Autodesk Inventor part; units mm, degrees
ref_plane "YZ Plane" through (0, 0, 0) normal (1, 0, 0) x (0, 1, 0)
ref_plane "XZ Plane" through (0, 0, 0) normal (0, 1, 0) x (-1, 0, 0)
ref_plane "XY Plane" through (0, 0, 0) normal (0, 0, 1) x (1, 0, 0)
sketch "Sketch1" plane through (0, 0, 0) normal (0, 1, 0) x (-1, 0, 0)
  line L0 (0, 0) -> (85.6, 0)
  line L1 (85.6, 0) -> (85.6, 53.98)
  line L2 (85.6, 53.98) -> (0, 53.98)
  line L3 (0, 53.98) -> (0, 0)
  line L4 (0, 53.98) -> (0, 50.8)
  line L5 (0, 50.8) -> (3.18, 50.8)
  circle A0 centre (3.18, 50.8) radius 3.18
  line L6 (85.6, 53.98) -> (85.6, 57.98)
  line L7 (85.6, 57.98) -> (0, 57.98)
  line L8 (0, 57.98) -> (-9, 57.98)
  line L9 (-9, 57.98) -> (-9, 0)
  line L10 (-9, 0) -> (0, 0)
  line L11 (0, 26.99) -> (-4.5, 26.99)
  circle A1 centre (-4.5, 26.99) radius 2.5
  line L12 (85.6, 55.98) -> (65.6, 55.98)
  circle A2 centre (65.6, 55.98) radius 1
  line L13 (0, 26.99) -> (85.6, 26.99)
  line L14 (85.6, -4) -> (0, -4)
  line L15 (0, -4) -> (-9, -4)
  circle A3 centre (65.6, -2) radius 1
  line L16 (85.6, -4) -> (85.6, 0)
  line L17 (-9, -4) -> (-9, 0)
  line L18 (85.6, 57.98) -> (88.6, 57.98)
  line L19 (88.6, 57.98) -> (88.6, -4)
  line L20 (88.6, -4) -> (85.6, -4)
  line L21 (85.6, -4) -> (85.6, 57.98)
  line L22 (85.6, 53.98) -> (88.6, 53.98)
  line L23 (85.6, 0) -> (88.6, 0)
  circle A4 centre (3.18, 3.18) radius 3.18
  point P0 (3.18, 0)
  point P1 (0, 3.18)
  point P2 (3.18, 53.98)
  dimension "d0" = 85.6
  dimension "d1" = 53.98
  dimension "d2" = 3.18
  dimension "d3" = 3.18
  dimension "d4" = 4
  dimension "d5" = 9
  dimension "d6" = 5
  dimension "d7" = 20
  dimension "d8" = 2
  dimension "d9" = 3
extrude "Extrusion1" add sketch "Sketch1" along normal blind 5 contours L3 A4 L0 | L10 L9 L8 L7 L6 L2 L3 | L0 L16 L14 L15 L17 L10 | L3 L2 A0 | L6 L18 L19 L22
extrude "Extrusion2" add sketch "Sketch1" along normal blind 1 contours A4 L3 L13 L1 L0 | A4 | L3 A0 L2 L1 L13 | A0
extrude "Extrusion3" add sketch "Sketch1" along normal blind 5 contours L23 L19 L20 L16
extrude "Extrusion4" add sketch "Sketch1" along normal blind 5 contours L1 L22 L19 L23
fillet "Fillet2" radius 4 4 edges at (-88.6, 2.5, 57.98) (-88.6, 2.5, -4) (9, 2.5, -4) (9, 2.5, 57.98)
extrude "Extrusion5" add sketch "Sketch1" along normal blind 3 contours A1 | A2 | A3
properties part number "magnet card bottom"
Geometry: final body of the model. Coordinates: model frame, mm. A direction names the side the tool comes from. Give positions to 0.01 mm unless a question says otherwise; leave off trailing zeros. Loops run counter-clockwise (first coordinate to the right, second up) from the corner with the lowest first, then second, coordinate; pieces in that order, holes last. Notation, with made-up numbers: (22, 87) - (50, 87) arc R21 cw to (50, 125) - close; hole circle Ø9 at (41.5, 34.5). An arc over 180 degrees is marked (long way). One line per question, with ' | ' between items. Start each with the question number.
(1) Section query B-B on x = -65.6. Return loops of the section in (y, z).
(2) Contact query for flat-ended pins moving along their axis: pin 1 (2.5 mm diameter, centred on x = 5, z = 26.5, fed in from +Y); pin 2 (5 mm diameter, centred on x = -37, z = 8, fed in from +Y). Output: stop coordinate, or through.
(3) Section query A-A on y = 2.2. Return loops of the section in (x, z).
(4) Pull-direction query (Z, two-part tool) for faces 1 (the cylindrical face through (-66.554, 3.986, 55.68)), 2 (the flat face through (9, 2, 27)), 3 (the cylindrical face through (7.797, 2.535, 56.839)); classes: released by +Z, released by -Z, zero draft, split by the parting line, or undercut.
(5) Section query D-D on x = -48. Return loops of the section in (y, z).
(6) Section query C-C on z = -2. Return loops of the section in (x, y), then the cut area to 3 significant figures.
(7) Ray query, line 1 (Z direction, x = -65.6, y = 4.45); line 2 (X direction, y = 4.45, z = 38.5); line 3 (Z direction, x = -23, y = 3.95). Return the intervals inside material, ascending. Write a range as from..to.
(8) Reachability of faces 4 (the cylindrical face through (-87.459, 2.535, 56.777)), 5 (the flat face through (-66, 3, 56)) from +Z, -Z, +X, -X, +Y, -Y: full face, straight path, thin tool, end or side. Return the list, or none.
The answers:
1) outline: (0, -4) - (5, -4) - (5, -3) - (3, -3) - (3, -1) - (5, -1) - (5, 0) - (1, 0) - (1, 53.98) - (5, 53.98) - (5, 54.98) - (3, 54.98) - (3, 56.98) - (5, 56.98) - (5, 57.98) - (0, 57.98) - close
2) pin 1: y = 3 | pin 2: y = 1
3) outline: (-88.6, 0) arc R4 ccw to (-84.6, -4) - (5, -4) arc R4 ccw to (9, 0) - (9, 53.98) arc R4 ccw to (5, 57.98) - (-84.6, 57.98) arc R4 ccw to (-88.6, 53.98) - close; hole (-85.6, 0) - (-3.18, 0) arc R3.18 ccw to (0, 3.18) - (0, 50.8) arc R3.18 ccw to (-3.18, 53.98) - (-85.6, 53.98) - close
4) face 1: undercut | face 2: zero draft | face 3: released by +Z
5) outline: (0, -4) - (5, -4) - (5, 0) - (1, 0) - (1, 53.98) - (5, 53.98) - (5, 57.98) - (0, 57.98) - close
6) outline: (-88.06, 0) - (8.46, 0) - (8.46, 5) - (-64.6, 5) - (-64.6, 3) - (-66.6, 3) - (-66.6, 5) - (-88.06, 5) - close | area: 479 mm2
7) line 1: -4..-3, -1..0, 53.98..54.98, 56.98..57.98 | line 2: -88.6..-85.6, 0..9 | line 3: -4..0, 53.98..57.98
8) face 4: +Z, -X, +Y, -Y | face 5: +Y
